```python
from build123d import *

# Parameters (mm, degrees)
SKETCH1_W                  = 63.5
SKETCH1_H                  = 19.05
SKETCH1_W_2                = 127
BOSS_EXTRUDE1_DEPTH        = 25.4
SKETCH5_R                  = 19.0627
CUT_EXTRUDE1_DEPTH         = 26.4
F_12_0_12_DIAMETER_HOLE1_D = 12


with BuildPart() as part:
    # Sketch1 → Boss-Extrude1 (new body)
    with BuildSketch(Plane.XY):
        with BuildLine():
            ThreePointArc((-31.75, 28.575), (0, 60.325), (31.75, 28.575))
            Line((31.75, 28.575), (-31.75, 28.575))
        make_face()
        with Locations((0, 19.05)):
            Rectangle(SKETCH1_W, SKETCH1_H)
        Rectangle(SKETCH1_W_2, SKETCH1_H)
    extrude(amount=BOSS_EXTRUDE1_DEPTH)

    # Sketch5 → Cut-Extrude1 (cut, through all)
    with BuildSketch(Plane(origin=(0, 0, 0), x_dir=(-1, 0, 0), z_dir=(0, 0, -1))):
        with Locations((0, 28.575)):
            Circle(SKETCH5_R)
    extrude(amount=-CUT_EXTRUDE1_DEPTH, mode=Mode.SUBTRACT)

    # Ø12.0 (12) Diameter Hole1 (through all)
    with Locations(Plane(origin=(0, 9.525, 0), x_dir=(1, 0, 0), z_dir=(0, 1, 0))):
        with Locations((-47.625, -12.7), (47.625, -12.7)):
            Hole(F_12_0_12_DIAMETER_HOLE1_D / 2)


solid = part.part
```
Source: CAD feature listing. Evaluate the final solid. Frame: model axes, mm. A direction names the side the tool comes from. Coordinates: 2 decimals unless noted, no trailing zeros. Loops run counter-clockwise (first coordinate to the right, second up) from the corner with the lowest first, then second, coordinate; pieces in that order, holes last. Notation, with made-up numbers: M 41,25 L 98,25 A12 cw 98,46 Z; hole C -19,1 d9. An arc over 180 degrees is marked long. Use a Markdown table: item, result. Add a question column.
Q1. Material intervals for L1, parallel to X at y = 2, z = 12.25; L2, parallel to Y at x = 38, z = 12.25 (3 decimals); L3, parallel to Y at x = 5, z = 12 (3 decimals), sorted ascending.
Q2. Draft query along Z for faces 1 (the cylindrical face through (-41.63, -0.13, 12.44)), 2 (the flat face through (1, 3, 0)), 3 (the flat face through (1, 3, 25.4)), 4 (the cylindrical face through (-0.698, 60.317, 12.522)). Return one class per face: pulls with the +Z half, pulls with the -Z half, needs draft (parallel to the pull), parting line crosses it, or undercut.
Q3. Section query C-C, the plane y = -2.5. Return loops of the section in (x, z) (3 decimals), and give its area (3 significant figures).
Q4. Section query A-A, the plane z = 12.7. Return loops of the section in (x, y) (3 decimals).
Q5. First-contact query: pin 1 (7 mm diameter, centred on x = -47.625, z = 12.7, fed in from -Y); pin 2 (9.5 mm diameter, centred on y = 23, z = 10, fed in from +X); pin 3 (12.5 mm diameter, centred on x = 54.5, z = 14, fed in from +Y) (3 decimals); pin 4 (10 mm diameter, centred on y = 49, z = 20.5, fed in from -X). Flat tips, straight axial feed; report the tip coordinate or a pass-through.
Q6. Access query for faces 5 (the flat face through (31.75, 19, 13)), 6 (the flat face through (-51, 9.525, 18)), 7 (the cylindrical face through (4.132, 9.966, 12.522)). Directions: +Z, -Z, +X, -X, +Y, -Y. A direction counts if a zero-diameter tool reaches every point of the face in a straight line with its end or side. Return the directions, or none.
Q7. Section query D-D, the plane y = 24.5. Return loops of the section in (x, z).
Q8. Section query B-B, the plane x = 0. Return loops of the section in (y, z) (3 decimals).
Result:
| question | item | result |
|---|---|---|
| 1 | L1 | x = -63.5 to -53.61, -41.64 to 41.64, 53.61 to 63.5 |
| 1 | L2 | y = -9.525 to 9.525 |
| 1 | L3 | y = -9.525 to 10.18, 46.97 to 59.929 |
| 2 | face 1 | undercut |
| 2 | face 2 | pulls with the -Z half |
| 2 | face 3 | pulls with the +Z half |
| 2 | face 4 | needs draft |
| 3 | outline | M -63.5,0 L 63.5,0 L 63.5,25.4 L -63.5,25.4 Z; hole C -47.625,12.7 d12; hole C 47.625,12.7 d12 |
| 3 | area | 3,000 mm2 |
| 4 | outline | M -63.5,-9.525 L -53.625,-9.525 L -53.625,9.525 L -63.5,9.525 Z; M -41.625,-9.525 L 41.625,-9.525 L 41.625,9.525 L 31.75,9.525 L 31.75,28.575 A31.75 ccw -31.75,28.575 L -31.75,9.525 L -41.625,9.525 Z; M 53.625,-9.525 L 63.5,-9.525 L 63.5,9.525 L 53.625,9.525 Z; hole C 0,28.575 d38.125 |
| 5 | pin 1 | passes through |
| 5 | pin 2 | stops at x = 31.75 |
| 5 | pin 3 | stops at y = 9.525 |
| 5 | pin 4 | stops at x = -27.75 |
| 6 | face 5 | +Z, -Z, +X, +Y |
| 6 | face 6 | +Z, -Z, -X, +Y |
| 6 | face 7 | +Z, -Z |
| 7 | outline | M -31.75,0 L -18.62,0 L -18.62,25.4 L -31.75,25.4 Z; M 18.62,0 L 31.75,0 L 31.75,25.4 L 18.62,25.4 Z |
| 8 | outline | M -9.525,0 L 9.512,0 L 9.512,25.4 L -9.525,25.4 Z; M 47.638,0 L 60.325,0 L 60.325,25.4 L 47.638,25.4 Z |
